Autodesk Inventor part; units mm, degrees
ref_plane "YZ Plane" through (0, 0, 0) normal (1, 0, 0) x (0, 1, 0)
ref_plane "XZ Plane" through (0, 0, 0) normal (0, 1, 0) x (-1, 0, 0)
ref_plane "XY Plane" through (0, 0, 0) normal (0, 0, 1) x (1, 0, 0)
sketch "Sketch1" plane through (0, 0, 0) normal (0, 0, 1) x (1, 0, 0)
  line L0 (0, 0) -> (0, 47.65)
  line L1 (47.65, 95.3) -> (95.3, 95.3)
  arc A0 (47.65, 95.3) -> (0, 47.65) centre (47.65, 47.65) ccw
  dimension "d0" = 95.3
  dimension "d1" = 95.3
  dimension "d2" = 47.65
sketch "Sketch2" plane through (0, 0, 0) normal (0, 1, 0) x (-1, 0, 0)
  circle A0 centre (0, 0) radius 19.05
  circle A1 centre (0, 0) radius 17.4
  dimension "d4" = 1.65
  dimension "d5" = 38.1
sweep "Sweep1" add profiles "Sketch2" path "Sketch1"
equation "\"d1\" = d0"
equation "\"d2\" = 0.5 * d0"
properties part number "ASME BPE 90DEG ELB-38.1"
Here's how the part is built. I have some questions about the finished solid (model axes, mm). A direction names the side the tool comes from. Round coordinates to 2 decimals unless told otherwise and drop trailing zeros. Write each loop counter-clockwise with the first axis right and the second up, starting at its lowest first coordinate (ties: lowest second). Pieces come first, ordered by that corner, then holes.
Q1. If we section it at D-D on z = 14: Write out the boundary of the cut face in (x, y).
Q2. If we section it at B-B on x = 72: Write out the boundary of the cut face in (y, z), plus the area to 3 significant figures.
Q3. Please list where these lines run through material, in increasing order: probe 1 along Y at (x, z) = (84, 0); probe 2 along Z at (x, y) = (0, 27); probe 3 along X at (y, z) = (54.5, -4).
Q4. If we section it at C-C on y = 35: Write out the boundary of the cut face in (x, z), plus the area to 3 significant figures.
Q5. If we section it at A-A on z = 0: Write out the boundary of the cut face in (x, y), plus the area to 3 significant figures.
Q6. If we mould it in two halves opening along Z, with no side actions, what happens to faces 4 (the cylindrical face through (71.8, 81.5, -10.6)), 5 (the cylindrical face through (15.12, 24.16, -11.59)), 6 (the flat face through (-15.43, 0, 8.38))? For each: +Z half, -Z half, draft (parallel to the pull), parting line (faces both ways), or undercut.
Q7. Which directions (+Z, -Z, +X, -X, +Y, -Y) give clear straight access to the entire face, cutting with the end or side of a thin tool? Please do faces 1 (the cylindrical face through (71.809, 91.17, -18.597)), 2 (the flat face through (95.3, 111, 8)), 3 (the cylindrical face through (3.772, 24.159, -16.986)).
Q8. Will these pins go through, and if not, where does the flat tip stop? P1, Ø1, axis at y = 101.5, z = 8, coming from the +X side; P2, Ø10, axis at y = 34.5, z = 7.5, coming from the -X side; P3, Ø6, axis at x = 45.5, z = -7.5, coming from the -Y side.
Answer below:
1. outline: (-12.92, 0) - (-10.33, 0) - (-10.33, 47.65) arc R57.98 cw to (47.65, 105.63) - (95.3, 105.63) - (95.3, 108.22) - (47.65, 108.22) arc R60.57 ccw to (-12.92, 47.65) - close; (10.33, 0) - (12.92, 0) - (12.92, 47.65) arc R34.73 cw to (47.65, 82.38) - (95.3, 82.38) - (95.3, 84.97) - (47.65, 84.97) arc R37.32 ccw to (10.33, 47.65) - close
2. outline: circle Ø38.1 at (95.3, 0); hole circle Ø34.8 at (95.3, 0)
2. area: 189 mm2
3. probe 1: y = 76.25 to 77.9, 112.7 to 114.35
3. probe 2: z = -19.05 to -17.4, 17.4 to 19.05
3. probe 3: x = -18.27 to -16.57, 17.71 to 19.45
4. outline: circle Ø38.1 at (0, 0); hole circle Ø34.8 at (0, 0)
4. area: 189 mm2
5. outline: (-19.05, 0) - (-17.4, 0) - (-17.4, 47.65) arc R65.05 cw to (47.65, 112.7) - (95.3, 112.7) - (95.3, 114.35) - (47.65, 114.35) arc R66.7 ccw to (-19.05, 47.65) - close; (17.4, 0) - (19.05, 0) - (19.05, 47.65) arc R28.6 cw to (47.65, 76.25) - (95.3, 76.25) - (95.3, 77.9) - (47.65, 77.9) arc R30.25 ccw to (17.4, 47.65) - close
5. area: 561 mm2
6. face 4: undercut
6. face 5: parting line
6. face 6: draft
7. face 1: +X
7. face 2: +Z, -Z, +X, +Y, -Y
7. face 3: -Y
8. P1: stops at x = 15.74
8. P2: stops at x = -18.89
8. P3: stops at y = 76.66
